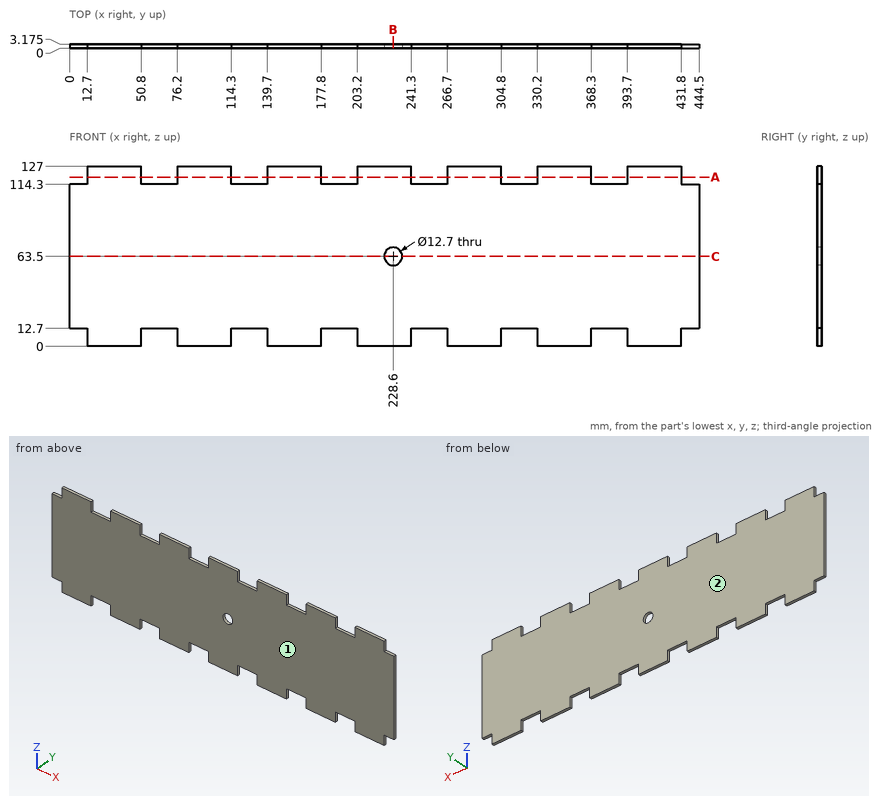
Geometry: see drawing. Coordinates: mm, zero at the bounding-box minimum. Give positions to 0.01 mm unless a question says otherwise; leave off trailing zeros. Order: outer loops, then holes, each group sorted by start corner. A loop starts at its lowest first (then second) coordinate and runs counter-clockwise, first axis right, second up. Notation, with made-up numbers: (-36.5, -15) - (9.5, -15) arc R31 cw to (9.5, 14) - close; hole circle Ø9 at (10, 8). An arc over 180 degrees is marked (long way). Use a Markdown table: item, result.
(1) Section query C-C (z = 63.5). Output: boundary loops of the cut face in (x, y) (3 decimals), then the cut area to 3 significant figures.
Computed values:
| item | result |
|---|---|
| outline | (0, 0) - (222.25, 0) - (222.25, 3.175) - (0, 3.175) - close; (234.95, 0) - (444.5, 0) - (444.5, 3.175) - (234.95, 3.175) - close |
| area | 1,370 mm2 |
(2) Line query: line 1 (X direction, y = 2, z = 63.5); line 2 (Z direction, x = 228.6, y = 2.05); line 3 (Z direction, x = 197, y = 2.1). Output: solid intervals per line, ascending. Write a range as from..to.
Computed values:
| item | result |
|---|---|
| line 1 | x = 0..222.25, 234.95..444.5 |
| line 2 | z = 0..57.15, 69.85..127 |
| line 3 | z = 12.7..114.3 |
(3) Section query A-A (z = 119.5). Output: boundary loops of the cut face in (x, y) (3 decimals), then the cut area to 3 significant figures.
Computed values:
| item | result |
|---|---|
| outline | (12.7, 0) - (50.8, 0) - (50.8, 3.175) - (12.7, 3.175) - close; (76.2, 0) - (114.3, 0) - (114.3, 3.175) - (76.2, 3.175) - close; (139.7, 0) - (177.8, 0) - (177.8, 3.175) - (139.7, 3.175) - close; (203.2, 0) - (241.3, 0) - (241.3, 3.175) - (203.2, 3.175) - close; (266.7, 0) - (304.8, 0) - (304.8, 3.175) - (266.7, 3.175) - close; (330.2, 0) - (368.3, 0) - (368.3, 3.175) - (330.2, 3.175) - close; (393.7, 0) - (431.8, 0) - (431.8, 3.175) - (393.7, 3.175) - close |
| area | 847 mm2 |
(4) Pin query (flat end, axial travel): pin 1 (1 mm diameter, centred on y = 2.5, z = 121.5, fed in from +X); pin 2 (1.5 mm diameter, centred on x = 255.5, y = 3, fed in from -Z); pin 3 (20.5 mm diameter, centred on x = 228.6, z = 63.5, fed in from -Y); pin 4 (1.6 mm diameter, centred on x = 196, y = 1.5, fed in from +Z). Return the tip coordinate at first contact, or that it passes through.
Computed values:
| item | result |
|---|---|
| pin 1 | stops at x = 431.8 |
| pin 2 | stops at z = 12.7 |
| pin 3 | stops at y = 0 |
| pin 4 | stops at z = 114.3 |
(5) Section query B-B (x = 228.6). Output: boundary loops of the cut face in (y, z) (3 decimals).
Computed values:
| item | result |
|---|---|
| outline | (0, 0) - (3.175, 0) - (3.175, 57.15) - (0, 57.15) - close; (0, 69.85) - (3.175, 69.85) - (3.175, 127) - (0, 127) - close |
(6) Draft query along Y for the marked faces 1 and 2. Return one class per face: released by +Y, released by -Y, zero draft, split by the parting line, or undercut.
Computed values:
| item | result |
|---|---|
| face 1 | released by -Y |
| face 2 | released by +Y |
